Verification items for the finished model (mm, model axes). A direction names the side the tool comes from. Round coordinates to 2 decimals unless told otherwise and drop trailing zeros. Order: outer loops, then holes, each group sorted by start corner. A loop starts at its lowest first (then second) coordinate and runs counter-clockwise, first axis right, second up. Notation, with made-up numbers: (0, 85) -> (14, 85) arc R14 ccw to (14, 105) -> close; hole circle Ø11 at (-30.5, -11.5). An arc over 180 degrees is marked (long way). Return JSON: item names as keys, results as strings. Group by question number.
1) Section check B-B on y = -2.5. Enter the section's corners in (x, z), plus the area to 3 significant figures.
2) Depth check by flat-ended pin: pin 1 (5 mm diameter, centred on y = 9.5, z = -8, fed in from -X); pin 2 (10 mm diameter, centred on x = -9, z = 5, fed in from +Y); pin 3 (12 mm diameter, centred on x = -23, z = 2, fed in from +Y). Enter the tip coordinate at first touch or a pass-through.
3) Section check C-C on z = -9.25. Enter the section's corners in (x, y).
4) Scan lines: L1, parallel to X at y = -6, z = 5; L2, parallel to X at y = 11.5, z = -4.25; L3, parallel to Y at x = -27, z = -0.75. Record each from-to range of solid material in increasing order.
5) Draft check along X on faces 6 (the flat face through (4, 15, -2)), 7 (the flat face through (16.5, 27.7, -7.3)), 8 (the flat face through (18, 18, 7)). Enter one of: pulls with the +X half, pulls with the -X half, needs draft (parallel to the pull), parting line crosses it, or undercut.
6) Section check A-A on x = 11. Enter the section's corners in (y, z), plus the area to 3 significant figures.
7) Tool access check on faces 1 (the flat face through (-18, 13, -5)), 2 (the flat face through (9, 15, -15)), 3 (the flat face through (26, 15, 5)), 4 (the flat face through (14.2, 15, -2)), 5 (the flat face through (11, 0, 5)). Record the directions out of +Z, -Z, +X, -X, +Y, -Y that give a thin tool (end or side, any length) a straight path to the whole face; none if there is none.
8) Section check D-D on x = -19. Enter the section's corners in (y, z), plus the area to 3 significant figures.
```python
from build123d import *

# Parameters (mm, degrees)
SZKIC1_W                        = 58
SZKIC1_H                        = 20
DODANIE_WYCI_GNI_CIE1_DEPTH     = 5
SZKIC2_W                        = 15
SZKIC2_H                        = 5
DODANIE_WYCI_GNI_CIE2_DEPTH     = 58
DODANIE_WYCI_GNI_CIE3_DEPTH     = 20
DODANIE_WYCI_GNI_CIE4_DEPTH     = 10
WYTNIJ_WYCI_GNI_CIE2_DEPTH      = 47.562216442
WYTNIJ_WYCI_GNI_CIE2_DEPTH_BACK = 47.562216442
SZKIC6_W                        = 58
SZKIC6_H                        = 5
DODANIE_WYCI_GNI_CIE5_DEPTH     = 20
SZKIC7_R                        = 2
WYTNIJ_WYCI_GNI_CIE3_DEPTH      = 10
DODANIE_WYCI_GNI_CIE8_DEPTH     = 10
SZKIC11_W                       = 10.2
SZKIC11_H                       = 10.2
DODANIE_WYCI_GNI_CIE9_DEPTH     = 5
SFAZOWANIE2_SIZE                = 5
SFAZOWANIE3_SIZE                = 5
SZKIC12_W                       = 10
SZKIC12_H                       = 20
WYTNIJ_WYCI_GNI_CIE4_DEPTH      = 10


with BuildPart() as part:
    # Szkic1 → Dodanie-wyciągnięcie1 (new body)
    with BuildSketch(Plane.XY):
        Rectangle(SZKIC1_W, SZKIC1_H)
    extrude(amount=DODANIE_WYCI_GNI_CIE1_DEPTH)

    # Szkic2 → Dodanie-wyciągnięcie2 (add)
    with BuildSketch(Plane(origin=(29, 0, 0), x_dir=(0, 0, -1), z_dir=(1, 0, 0))):
        with Locations((-2.5, 12.5)):
            Rectangle(SZKIC2_W, SZKIC2_H)
    extrude(amount=-DODANIE_WYCI_GNI_CIE2_DEPTH)

    # Szkic3 → Dodanie-wyciągnięcie3 (add)
    with BuildSketch(Plane.XZ.offset(10)):
        Polygon((-34, 5), (-29, 0), (-29, 5), (-24, 5), (-29, 10), (-34, 10), align=None)
    extrude(amount=-DODANIE_WYCI_GNI_CIE3_DEPTH)

    # Szkic5 → Dodanie-wyciągnięcie4 (add)
    with BuildSketch(Plane.XY.offset(5)):
        Polygon((14.2, 20.2), (14.2, 10), (19, 10), (19, 30.2), (-6, 30.2), (-6, 10), (4, 10), (4, 20.2), align=None)
    extrude(amount=-DODANIE_WYCI_GNI_CIE4_DEPTH)

    # Szkic5<3> → Wytnij-wyciągnięcie2 (cut, two sides: drawn at the far end of the back side and taken through both)
    with BuildSketch(Plane.XY.offset(5).offset(-WYTNIJ_WYCI_GNI_CIE2_DEPTH_BACK)):
        Polygon((4, 10), (14.2, 10), (14.2, 15), (14.2, 20.2), (4, 20.2), (4, 15), align=None)
    extrude(amount=WYTNIJ_WYCI_GNI_CIE2_DEPTH + WYTNIJ_WYCI_GNI_CIE2_DEPTH_BACK, mode=Mode.SUBTRACT)

    # Szkic6 → Dodanie-wyciągnięcie5 (add)
    with BuildSketch(Plane(origin=(0, 10, 0), x_dir=(1, 0, 0), z_dir=(0, 1, 0))):
        with Locations((0, -7.5)):
            Rectangle(SZKIC6_W, SZKIC6_H)
    extrude(amount=-DODANIE_WYCI_GNI_CIE5_DEPTH)

    # Szkic7 → Wytnij-wyciągnięcie3 (cut)
    with BuildSketch(Plane.XZ.offset(10)):
        with Locations(Location((-19, 5, 0), (0, 0, 270))):
            Circle(SZKIC7_R)
        with Locations(Location((11, 5, 0), (0, 0, 270))):
            Circle(SZKIC7_R)
    extrude(amount=-WYTNIJ_WYCI_GNI_CIE3_DEPTH, mode=Mode.SUBTRACT)

    # Szkic10 → Dodanie-wyciągnięcie8 (add)
    with BuildSketch(Plane(origin=(0, 0, -5), x_dir=(-1, 0, 0), z_dir=(0, 0, -1))):
        Polygon((6, 10), (6, 15), (6, 30.2), (-19, 30.2), (-19, 15), (-29, 15), (-29, 10), (-14.2, 10), (-14.2, 20.2), (-4, 20.2), (-4, 10), align=None)
    extrude(amount=DODANIE_WYCI_GNI_CIE8_DEPTH)

    # Szkic11 → Dodanie-wyciągnięcie9 (add)
    with BuildSketch(Plane(origin=(0, 0, -15), x_dir=(-1, 0, 0), z_dir=(0, 0, -1))):
        with Locations((-9.1, 15.1)):
            Rectangle(SZKIC11_W, SZKIC11_H)
        Polygon((-29, 10), (-14.2, 10), (-14.2, 20.2), (-4, 20.2), (-4, 10), (6, 10), (6, 30.2), (-19, 30.2), (-19, 15), (-29, 15), align=None)
    extrude(amount=DODANIE_WYCI_GNI_CIE9_DEPTH)

    # Sfazowanie2
    sfazowanie2_edges = [part.edges().sort_by_distance(p)[0] for p in [
        (-6, 30.2, -7.5),
        (19, 30.2, -7.5),
    ]]
    chamfer(sfazowanie2_edges, length=SFAZOWANIE2_SIZE)

    # Sfazowanie3
    # the kernel refuses this chamfer: 5 mm, written as the material it adds along each edge
    with BuildSketch(Plane(origin=(1.34158506, 15, 5), x_dir=(0, 0.9996219169112968, -0.027495876610586317), z_dir=(1, 0, 0))) as sfazowanie3_piece_1_section:
        Polygon((SFAZOWANIE3_SIZE * 0.999621916911, SFAZOWANIE3_SIZE * 0.0274958766106), (-SFAZOWANIE3_SIZE * 0.0274958766106, SFAZOWANIE3_SIZE * 0.999621916911), (0, 0), align=None)
    sfazowanie3_piece_1 = extrude(amount=17.65841494, mode=Mode.PRIVATE)
    sfazowanie3_piece_1 = split(sfazowanie3_piece_1, bisect_by=Plane(origin=(4, 16.652020772, 6.643171669), z_dir=(-1, 0, 0)), keep=Keep.TOP, mode=Mode.PRIVATE)
    sfazowanie3_piece_1 = split(sfazowanie3_piece_1, bisect_by=Plane(origin=(2.67079253, 16.652020772, 10), z_dir=(0, 0, -1)), keep=Keep.TOP, mode=Mode.PRIVATE)
    add(sfazowanie3_piece_1)
    with BuildSketch(Plane(origin=(14.2, 15, 5), x_dir=(0, 0.9996219169112968, -0.027495876610586317), z_dir=(1, 0, 0))) as sfazowanie3_piece_2_section:
        Polygon((SFAZOWANIE3_SIZE * 0.999621916911, SFAZOWANIE3_SIZE * 0.0274958766106), (-SFAZOWANIE3_SIZE * 0.0274958766106, SFAZOWANIE3_SIZE * 0.999621916911), (0, 0), align=None)
    sfazowanie3_piece_2 = extrude(amount=4.8, mode=Mode.PRIVATE)
    sfazowanie3_piece_2 = split(sfazowanie3_piece_2, bisect_by=Plane(origin=(16.6, 16.652020772, 10), z_dir=(0, 0, -1)), keep=Keep.TOP, mode=Mode.PRIVATE)
    add(sfazowanie3_piece_2)
    with BuildSketch(Plane(origin=(-6, 15, 5), x_dir=(0, 0.9996219169112968, -0.027495876610586317), z_dir=(1, 0, 0))) as sfazowanie3_piece_3_section:
        Polygon((SFAZOWANIE3_SIZE * 0.999621916911, SFAZOWANIE3_SIZE * 0.0274958766106), (-SFAZOWANIE3_SIZE * 0.0274958766106, SFAZOWANIE3_SIZE * 0.999621916911), (0, 0), align=None)
    sfazowanie3_piece_3 = extrude(amount=10, mode=Mode.PRIVATE)
    sfazowanie3_piece_3 = split(sfazowanie3_piece_3, bisect_by=Plane(origin=(-1, 16.652020772, 10), z_dir=(0, 0, -1)), keep=Keep.TOP, mode=Mode.PRIVATE)
    add(sfazowanie3_piece_3)
    with BuildSketch(Plane(origin=(-6, 15, 5), x_dir=(0, 0.9996219169112968, -0.027495876610586317), z_dir=(1, 0, 0))) as sfazowanie3_piece_4_section:
        Polygon((SFAZOWANIE3_SIZE * 0.999621916911, SFAZOWANIE3_SIZE * 0.0274958766106), (-SFAZOWANIE3_SIZE * 0.0274958766106, SFAZOWANIE3_SIZE * 0.999621916911), (0, 0), align=None)
    sfazowanie3_piece_4 = extrude(amount=22.85841494, mode=Mode.PRIVATE)
    sfazowanie3_piece_4 = split(sfazowanie3_piece_4, bisect_by=Plane(origin=(14.2, 16.652020772, 6.643171669), z_dir=(1, 0, 0)), keep=Keep.TOP, mode=Mode.PRIVATE)
    sfazowanie3_piece_4 = split(sfazowanie3_piece_4, bisect_by=Plane(origin=(15.52920747, 16.652020772, 10), z_dir=(0, 0, -1)), keep=Keep.TOP, mode=Mode.PRIVATE)
    add(sfazowanie3_piece_4)
    with BuildSketch(Plane(origin=(-6, 15, -5), x_dir=(0.027495876610586837, 0.9996219169112968, 0), z_dir=(0, 0, 1))) as sfazowanie3_piece_5:
        Polygon((SFAZOWANIE3_SIZE * 0.999621916911, SFAZOWANIE3_SIZE * 0.0274958766106), (-SFAZOWANIE3_SIZE * 0.0274958766106, SFAZOWANIE3_SIZE * 0.999621916911), (0, 0), align=None)
    extrude(amount=10)
    with BuildSketch(Plane(origin=(19, 15, -20), x_dir=(0.9996219169112968, -0.027495876610586664, 0), z_dir=(0, 0, 1))) as sfazowanie3_piece_6:
        Polygon((SFAZOWANIE3_SIZE * 0.999621916911, SFAZOWANIE3_SIZE * 0.0274958766106), (-SFAZOWANIE3_SIZE * 0.0274958766106, SFAZOWANIE3_SIZE * 0.999621916911), (0, 0), align=None)
    extrude(amount=25)
    with BuildSketch(Plane(origin=(14.2, 15, 5), x_dir=(0, 0.9996219169112968, -0.027495876610586317), z_dir=(1, 0, 0))) as sfazowanie3_piece_7a_section:
        Polygon((SFAZOWANIE3_SIZE * 0.999621916911, SFAZOWANIE3_SIZE * 0.0274958766106), (-SFAZOWANIE3_SIZE * 0.0274958766106, SFAZOWANIE3_SIZE * 0.999621916911), (0, 0), align=None)
    sfazowanie3_piece_7a = extrude(amount=17.65841494, mode=Mode.PRIVATE)
    sfazowanie3_piece_7a = split(sfazowanie3_piece_7a, bisect_by=Plane(origin=(19, 16.652020772, 6.643171669), z_dir=(1, 0, 0)), keep=Keep.TOP, mode=Mode.PRIVATE)
    sfazowanie3_piece_7a = split(sfazowanie3_piece_7a, bisect_by=Plane(origin=(24, 16.652020772, 10), z_dir=(0, 0, -1)), keep=Keep.TOP, mode=Mode.PRIVATE)
    sfazowanie3_piece_7a = split(sfazowanie3_piece_7a, bisect_by=Plane(origin=(29, 16.652020772, 6.643171669), z_dir=(-1, 0, 0)), keep=Keep.TOP, mode=Mode.PRIVATE)
    with BuildSketch(Plane(origin=(19, 15, -20), x_dir=(0.9996219169112968, -0.027495876610586664, 0), z_dir=(0, 0, 1))) as sfazowanie3_piece_7b_section:
        Polygon((SFAZOWANIE3_SIZE * 0.999621916911, SFAZOWANIE3_SIZE * 0.0274958766106), (-SFAZOWANIE3_SIZE * 0.0274958766106, SFAZOWANIE3_SIZE * 0.999621916911), (0, 0), align=None)
    sfazowanie3_piece_7b = extrude(amount=37.85841494, mode=Mode.PRIVATE)
    sfazowanie3_piece_7b = split(sfazowanie3_piece_7b, bisect_by=Plane(origin=(20.648968134, 16.648968134, 5), z_dir=(0, 0, 1)), keep=Keep.TOP, mode=Mode.PRIVATE)
    sfazowanie3_piece_7b = split(sfazowanie3_piece_7b, bisect_by=Plane(origin=(20.648968134, 16.648968134, 10), z_dir=(0, 0, -1)), keep=Keep.TOP, mode=Mode.PRIVATE)
    sfazowanie3_piece_7 = sfazowanie3_piece_7a & sfazowanie3_piece_7b
    add(sfazowanie3_piece_7)
    with BuildSketch(Plane(origin=(-6, 15, -5), x_dir=(0.027495876610586837, 0.9996219169112968, 0), z_dir=(0, 0, 1))) as sfazowanie3_piece_8a_section:
        Polygon((SFAZOWANIE3_SIZE * 0.999621916911, SFAZOWANIE3_SIZE * 0.0274958766106), (-SFAZOWANIE3_SIZE * 0.0274958766106, SFAZOWANIE3_SIZE * 0.999621916911), (0, 0), align=None)
    sfazowanie3_piece_8a = extrude(amount=22.85841494, mode=Mode.PRIVATE)
    sfazowanie3_piece_8a = split(sfazowanie3_piece_8a, bisect_by=Plane(origin=(-7.648968134, 16.648968134, 5), z_dir=(0, 0, 1)), keep=Keep.TOP, mode=Mode.PRIVATE)
    sfazowanie3_piece_8a = split(sfazowanie3_piece_8a, bisect_by=Plane(origin=(-7.648968134, 16.648968134, 10), z_dir=(0, 0, -1)), keep=Keep.TOP, mode=Mode.PRIVATE)
    with BuildSketch(Plane(origin=(-18.85841494, 15, 5), x_dir=(0, 0.9996219169112968, -0.027495876610586317), z_dir=(1, 0, 0))) as sfazowanie3_piece_8b_section:
        Polygon((SFAZOWANIE3_SIZE * 0.999621916911, SFAZOWANIE3_SIZE * 0.0274958766106), (-SFAZOWANIE3_SIZE * 0.0274958766106, SFAZOWANIE3_SIZE * 0.999621916911), (0, 0), align=None)
    sfazowanie3_piece_8b = extrude(amount=22.85841494, mode=Mode.PRIVATE)
    sfazowanie3_piece_8b = split(sfazowanie3_piece_8b, bisect_by=Plane(origin=(-6, 16.652020772, 6.643171669), z_dir=(-1, 0, 0)), keep=Keep.TOP, mode=Mode.PRIVATE)
    sfazowanie3_piece_8b = split(sfazowanie3_piece_8b, bisect_by=Plane(origin=(-12.42920747, 16.652020772, 10), z_dir=(0, 0, -1)), keep=Keep.TOP, mode=Mode.PRIVATE)
    sfazowanie3_piece_8 = sfazowanie3_piece_8a & sfazowanie3_piece_8b
    add(sfazowanie3_piece_8)

    # Szkic12 → Wytnij-wyciągnięcie4 (cut)
    with BuildSketch(Plane.XZ.offset(-10)):
        with Locations((24, -10)):
            Rectangle(SZKIC12_W, SZKIC12_H)
    extrude(amount=-WYTNIJ_WYCI_GNI_CIE4_DEPTH, mode=Mode.SUBTRACT)


solid = part.part
```
Check result:
{
 "1": {"outline": "(-34, 5) -> (-29, 0) -> (29, 0) -> (29, 10) -> (-34, 10) -> close; hole circle Ø4 at (-19, 5); hole circle Ø4 at (11, 5)", "area": "592 mm^2"},
 "2": {"pin 1": "x = -6", "pin 2": "y = 27.2", "pin 3": "y = 15"},
 "3": {"outline": "(-6, 10) -> (4, 10) -> (4, 20.2) -> (14.2, 20.2) -> (14.2, 10) -> (19, 10) -> (19, 25.2) -> (14, 30.2) -> (-1, 30.2) -> (-6, 25.2) -> close"},
 "4": {"L1": "-34 to -21, -17 to 9, 13 to 29", "L2": "-29 to 4, 14.2 to 19", "L3": "10 to 15"},
 "5": {"face 6": "undercut", "face 7": "pulls with the +X half", "face 8": "needs draft"},
 "6": {"outline": "(-10, 0) -> (10, 0) -> (10, 10) -> (-10, 10) -> (-10, 7) -> (0, 7) -> (0, 3) -> (-10, 3) -> close; (10, -20) -> (30.2, -20) -> (30.2, 5) -> (20.2, 5) -> (20.2, -15) -> (10, -15) -> close", "area": "461 mm^2"},
 "7": {"face 1": "-Z, -X, +Y, -Y", "face 2": "+Z, -Y", "face 3": "+Z, -Z, +X, +Y", "face 4": "+Z", "face 5": "-Y"},
 "8": {"outline": "(-10, 0) -> (10, 0) -> (10, -5) -> (15, -5) -> (15, 10) -> (-10, 10) -> (-10, 7) -> (0, 7) -> (0, 3) -> (-10, 3) -> close", "area": "235 mm^2"}
}
